from build123d import *

# Parameters (mm, degrees)
PAD016_DEPTH         = 27.5
POCKET034_DEPTH      = 185.628421
SKETCH105_W          = 70
SKETCH105_H          = 70
POCKET036_DEPTH      = 2.501
POCKET050_DEPTH      = 22.501
SKETCH114_W          = 70
SKETCH114_H          = 16
POCKET051_DEPTH      = 30.601
POCKET051_DEPTH_BACK = 30.601
PAD020_DEPTH         = 5
SKETCH134_R          = 2.3
SKETCH135_R          = 4
POCKET052_DEPTH      = 9


with BuildPart() as part:
    # Sketch096 → Pad016 (new body)
    with BuildSketch(Plane.XY.offset(2.5)):
        with BuildLine():
            Line((-22.6, 30.6), (22.6, 30.6))
            ThreePointArc((30.6, 22.6), (28.256854, 28.256854), (22.6, 30.6))
            Line((30.6, 22.6), (30.6, -22.6))
            ThreePointArc((22.6, -30.6), (28.256854, -28.256854), (30.6, -22.6))
            Line((22.6, -30.6), (-22.6, -30.6))
            ThreePointArc((-30.6, -22.6), (-28.256854, -28.256854), (-22.6, -30.6))
            Line((-30.6, -22.6), (-30.6, 22.6))
            ThreePointArc((-22.6, 30.6), (-28.256854, 28.256854), (-30.6, 22.6))
        make_face()
    extrude(amount=-PAD016_DEPTH)

    # Sketch103 → Pocket034 (cut, through all)
    with BuildSketch(Plane.XY.offset(-1.5)):
        with BuildLine():
            Line((14.1, 7.65), (20.4, 7.65))
            ThreePointArc((21.9, 6.15), (21.46066, 7.21066), (20.4, 7.65))
            Line((21.9, 6.15), (21.9, -6.15))
            ThreePointArc((20.4, -7.65), (21.46066, -7.21066), (21.9, -6.15))
            Line((20.4, -7.65), (14.1, -7.65))
            ThreePointArc((12.6, -6.15), (13.03934, -7.21066), (14.1, -7.65))
            Line((12.6, -6.15), (12.6, 6.15))
            ThreePointArc((14.1, 7.65), (13.03934, 7.21066), (12.6, 6.15))
        make_face()
    pocket034 = extrude(amount=POCKET034_DEPTH, mode=Mode.SUBTRACT)

    # Mirrored008: Pocket034 across YZ
    add(pocket034.mirror(Plane.YZ), mode=Mode.SUBTRACT)

    # Sketch105 → Pocket036 (cut, through all)
    with BuildSketch(Plane.XY):
        Rectangle(SKETCH105_W, SKETCH105_H)
        with BuildLine():
            Line((-22.8, 25.9), (22.8, 25.9))
            ThreePointArc((26.3, 22.4), (25.274874, 24.874874), (22.8, 25.9))
            Line((26.3, 22.4), (26.3, -22.4))
            ThreePointArc((22.8, -25.9), (25.274874, -24.874874), (26.3, -22.4))
            Line((22.8, -25.9), (-22.8, -25.9))
            ThreePointArc((-26.3, -22.4), (-25.274874, -24.874874), (-22.8, -25.9))
            Line((-26.3, -22.4), (-26.3, 22.4))
            ThreePointArc((-22.8, 25.9), (-25.274874, 24.874874), (-26.3, 22.4))
        make_face(mode=Mode.SUBTRACT)
    extrude(amount=POCKET036_DEPTH, mode=Mode.SUBTRACT)

    # Sketch107 → Groove012 (revolve, cut)
    with BuildSketch(Plane.XZ):
        Polygon((19, -1.5), (21.8, -1.5), (21.2, -3.148486), (21.2, -13.5), (19, -13.5), align=None)
    groove012 = revolve(axis=Axis((19, 0, -1.5), (0, 0, 1)), mode=Mode.SUBTRACT)

    # Mirrored009: Groove012 across YZ
    add(groove012.mirror(Plane.YZ), mode=Mode.SUBTRACT)

    # Sketch113 → Pocket050 (cut, through all)
    with BuildSketch(Plane.XY.offset(-20)):
        with BuildLine():
            ThreePointArc((22.834936, 22.25), (23.854356, 21.692811), (25, 21.5))
            ThreePointArc((27, 19.5), (26.414214, 20.914214), (25, 21.5))
            Line((27, 9.5), (27, 19.5))
            ThreePointArc((23.5, 6), (25.974874, 7.025126), (27, 9.5))
            Line((9.5, 6), (23.5, 6))
            ThreePointArc((6, 9.5), (7.025126, 7.025126), (9.5, 6))
            Line((6, 19.5), (6, 9.5))
            ThreePointArc((9.5, 23), (7.025126, 21.974874), (6, 19.5))
            Line((20.669873, 23), (9.5, 23))
            ThreePointArc((22.834936, 22.25), (21.815517, 22.807189), (20.669873, 23))
        make_face()
    extrude(amount=POCKET050_DEPTH, mode=Mode.SUBTRACT)

    # Sketch114 → Pocket051 (cut, two sides)
    with BuildSketch(Plane.XZ) as pocket051_sk:
        with Locations((0, -18)):
            Rectangle(SKETCH114_W, SKETCH114_H)
    extrude(amount=-POCKET051_DEPTH, mode=Mode.SUBTRACT)
    extrude(pocket051_sk.sketch, amount=POCKET051_DEPTH_BACK, mode=Mode.SUBTRACT)

    # AdditivePipe004: sweep along a path in Sketch130
    with BuildLine(Plane.XY) as additivepipe004_path:
        Line((24, 16), (24, 0))
        ThreePointArc((24, 0), (22.68034, -5.59017), (19, -10))
        ThreePointArc((19, -10), (15.31966, -14.40983), (14, -20))
        Line((14, -20), (14, -30.6))
    # Sketch131 → AdditivePipe004 (sweep)
    with BuildSketch(Plane.XZ):
        with BuildLine():
            ThreePointArc((26.037037, -18.550697), (24, -17.5), (21.962963, -18.550697))
            ThreePointArc((21.6, -18.434752), (21.739142, -18.625268), (21.962963, -18.550697))
            Line((21.6, -10), (21.6, -18.434752))
            Line((26.4, -10), (21.6, -10))
            Line((26.4, -18.434752), (26.4, -10))
            ThreePointArc((26.037037, -18.550697), (26.260858, -18.625268), (26.4, -18.434752))
        make_face()
    sweep(path=additivepipe004_path.line)

    # Sketch110 → Pad020 (join)
    with BuildSketch(Plane.XZ.offset(30.6)):
        with BuildLine():
            ThreePointArc((-8.85, -18.1), (-9.422826, -18.213685), (-9.908824, -18.537506))
            ThreePointArc((-10.25, -18.395841), (-10.126696, -18.58055), (-9.908824, -18.537506))
            Line((-10.25, -10), (-10.25, -18.395841))
            Line((-2.25, -10), (-10.25, -10))
            Line((-2.25, -18.395841), (-2.25, -10))
            ThreePointArc((-2.591176, -18.537506), (-2.373304, -18.58055), (-2.25, -18.395841))
            ThreePointArc((-2.591176, -18.537506), (-3.077174, -18.213685), (-3.65, -18.1))
            Line((-8.85, -18.1), (-3.65, -18.1))
        make_face()
    extrude(amount=-PAD020_DEPTH)

    # Sketch134 → AdditiveLoft section 0
    with BuildSketch(Plane.XY.offset(-17.5)):
        with Locations((-6, -6.5)):
            Circle(SKETCH134_R)
    # Sketch135 → AdditiveLoft section 1
    with BuildSketch(Plane.XY.offset(-10)):
        with Locations((-6, -6.5)):
            Circle(SKETCH135_R)
    loft()

    # AdditivePipe005: sweep along a path in Sketch136
    with BuildLine(Plane.XY) as additivepipe005_path:
        Line((-22.5, 27.5), (22.5, 27.5))
        ThreePointArc((22.5, 27.5), (26.035534, 26.035534), (27.5, 22.5))
        Line((27.5, 22.5), (27.5, -22.5))
        ThreePointArc((27.5, -22.5), (26.035534, -26.035534), (22.5, -27.5))
        Line((22.5, -27.5), (-22.5, -27.5))
        ThreePointArc((-22.5, -27.5), (-26.035534, -26.035534), (-27.5, -22.5))
        Line((-27.5, -22.5), (-27.5, 22.5))
        ThreePointArc((-27.5, 22.5), (-26.035534, 26.035534), (-22.5, 27.5))
    # Sketch137 → AdditivePipe005 (sweep)
    with BuildSketch(Plane.YZ):
        Polygon((28.397056, -10), (26.602944, -10), (27.1, -11.2), (27.9, -11.2), align=None)
    sweep(path=additivepipe005_path.line)

    # Sketch104 → Pocket052 (cut, symmetric)
    with BuildSketch(Plane.XY.offset(-11)):
        Polygon((-26.5, 27), (17.5, 27), (17.5, 23), (15.5, 23), (15.5, 7), (-25.5, 7), (-25.5, 23), (-26.5, 23), align=None)
    extrude(amount=POCKET052_DEPTH, both=True, mode=Mode.SUBTRACT)

    # Sketch099 → Groove018 (revolve, cut)
    with BuildSketch(Plane.XZ.offset(6)):
        Polygon((-26, 3), (-26, -24), (-24.2, -24), (-24.2, -8), (-23, -6.8), (-23, 3), align=None)
    revolve(axis=Axis((-26, -6, 3), (0, 0, 1)), mode=Mode.SUBTRACT)

    # Sketch100 → Groove019 (revolve, cut)
    with BuildSketch(Plane.XZ.offset(25)):
        Polygon((25, 3), (25, -24), (26.8, -24), (26.8, -8), (28, -6.8), (28, 3), align=None)
    revolve(axis=Axis((25, -25, 3), (0, 0, 1)), mode=Mode.SUBTRACT)

    # Sketch101 → Groove020 (revolve, cut)
    with BuildSketch(Plane.XZ.offset(-25)):
        Polygon((25, 3), (25, -24), (26.8, -24), (26.8, -8), (28, -6.8), (28, 3), align=None)
    revolve(axis=Axis((25, 25, 3), (0, 0, 1)), mode=Mode.SUBTRACT)


solid = part.part
Build history of the part. All positions in model axes, mm. A direction names the side the tool comes from. Give positions to 0.01 mm unless a question says otherwise; leave off trailing zeros. Order: outer loops, then holes, each group sorted by start corner. A loop starts at its lowest first (then second) coordinate and runs counter-clockwise, first axis right, second up. Notation, with made-up numbers: M 58,23.5 L 90,23.5 A7 ccw 90,34.5 Z; hole C -25.75,19 d10. An arc over 180 degrees is marked long. Put each result on its own line as item: value.
Item 1: Slice it at B-B, the plane y = 14. Write the cut outline in (x, z), plus the area to 3 significant figures.
From the geometry:
outline: M -30.6,-10 L -28.4,-10 L -27.9,-11.2 L -27.1,-11.2 L -26.6,-10 L -25.5,-10 L -25.5,-2 L 6,-2 L 6,2.5 L -26.3,2.5 L -26.3,0 L -30.6,0 Z; M 21.6,-18.43 A0.2 ccw 21.96,-18.55 A2.5 cw 26.04,-18.55 A0.2 ccw 26.4,-18.43 L 26.4,-10 L 21.6,-10 Z; M 26.6,-10 L 27.1,-11.2 L 27.9,-11.2 L 28.4,-10 L 30.6,-10 L 30.6,0 L 27,0 L 27,-10 Z
area: 272 mm2
Item 2: Slice it at C-C, the plane z = -14.75. Write the cut outline in (x, y).
From the geometry:
outline: M -10.25,-30.6 L -2.25,-30.6 L -2.25,-25.6 L -10.25,-25.6 Z; C -6,-6.5 d5.85; M 11.6,-30.6 L 16.4,-30.6 L 16.4,-20 A10.1 cw 20.44,-11.92 A14.9 ccw 26.4,0 L 26.4,16 L 21.6,16 L 21.6,0 A10.1 cw 17.56,-8.08 A14.9 ccw 11.6,-20 Z
Item 3: Slice it at A-A, the plane x = 10.5. Write the cut outline in (y, z), plus the area to 3 significant figures.
From the geometry:
outline: M -30.6,-10 L -28.4,-10 L -27.9,-11.2 L -27.1,-11.2 L -26.6,-10 L 6,-10 L 6,2.5 L -25.9,2.5 L -25.9,0 L -30.6,0 Z; M 23,-2 L 27,-2 L 27,-10.96 L 27.1,-11.2 L 27.9,-11.2 L 28.4,-10 L 30.6,-10 L 30.6,0 L 25.9,0 L 25.9,2.5 L 23,2.5 Z
area: 500 mm2
Item 4: Slice it at D-D, the plane x = -6. Write the cut outline in (y, z).
From the geometry:
outline: M -30.6,-18.1 L -25.6,-18.1 L -25.6,-10 L -10.5,-10 L -8.8,-17.5 L -4.2,-17.5 L -2.5,-10 L 7,-10 L 7,-2 L 27,-2 L 27,-10.96 L 27.1,-11.2 L 27.9,-11.2 L 28.4,-10 L 30.6,-10 L 30.6,0 L 25.9,0 L 25.9,2.5 L -25.9,2.5 L -25.9,0 L -30.6,0 Z
Item 5: 3-axis set-ups, long thin cutter, end or side, ignore diameter. For faces 1 (the flat face through (-26.3, 10, 1)), 2 (the flat face through (22, 24, -10)), 3 (the cylindrical face through (26.43, 20.9, -3.84)): which of +Z, -Z, +X, -X, +Y, -Y reach the whole face in a straight line?
From the geometry:
face 1: +Z, -X, +Y, -Y
face 2: -Z
face 3: +Z
Item 6: Probe line 1 (Y direction, x = -19, z = -7); line 2 (Y direction, x = -6, z = -5); line 3 (X direction, y = -6, z = -0.75). List the from-to ranges inside material, lowest first. Write a range as [from, to].
From the geometry:
line 1: y = [-30.6, -2.2], [2.2, 7], [27, 30.6]
line 2: y = [-30.6, 7], [27, 30.6]
line 3: x = [-30.6, -29], [-23, -21.9], [-12.6, 12.6], [21.9, 30.6]
Item 7: Flat gauge pins, fed straight in: pin 1 Ø2 at (y, z) = (-15.5, 1.5) entering from -X; pin 2 Ø10 at (x, y) = (-19.5, 17) entering from -Z; pin 3 Ø4.5 at (x, y) = (-26, -6) entering from +Z. Where does each tip first touch, or does it go through?
From the geometry:
pin 1: stops at x = -26.3
pin 2: stops at z = -2
pin 3: stops at z = -7.55
Item 8: Two-plate mould, pull along Y, no slides. Class faces 4 (the cylindrical face through (14, -25.4, -17.5)), 5 (the flat face through (-21.9, 0, 0)), 6 (the flat face through (0, 30.6, -5)): +Y half, -Y half, draft (parallel to the pull), parting line (faces both ways), or undercut.
From the geometry:
face 4: draft
face 5: undercut
face 6: +Y half
